For this review, take the finished solid that the model builds, in its own axes (mm). Face numbers are marked on the shaded views. A direction names the side the tool comes from. Round coordinates to 2 decimals unless told otherwise and drop trailing zeros. Order: outer loops, then holes, each group sorted by start corner. A loop starts at its lowest first (then second) coordinate and runs counter-clockwise, first axis right, second up. Notation, with made-up numbers: M 48.25,-11.5 L 104.25,-11.5 A25 cw 104.25,3.5 Z; hole C 18.25,24 d8. An arc over 180 degrees is marked long. Answer as a JSON object with one key per item and string values.
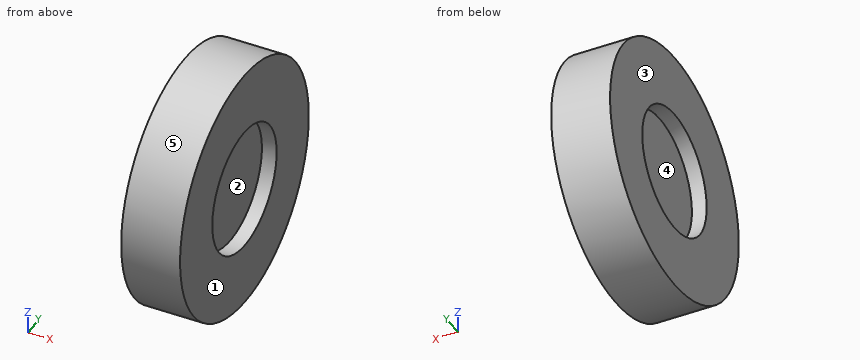
from build123d import *

# Parameters (mm, degrees)
SKETCH_1_W = 3
SKETCH_1_H = 6.35
SKETCH_4_W = 6
SKETCH_4_H = 6.35


with BuildPart() as part:
    # 草图1 → 旋转2 (revolve)
    with BuildSketch(Plane.XY, mode=Mode.PRIVATE) as revolve_2_sk:
        with Locations((0, 3.175)):
            Rectangle(SKETCH_1_W, SKETCH_1_H)
    revolve(revolve_2_sk.sketch.rotate(Axis((-1.5, 0, 0), (1, 0, 0)), 90), axis=Axis((-1.5, 0, 0), (1, 0, 0)))  # turned: the seam where the file's is

    # 草图4 → 旋转3 (revolve)
    with BuildSketch(Plane.XY, mode=Mode.PRIVATE) as revolve_3_sk:
        with Locations((0, 9.525)):
            Rectangle(SKETCH_4_W, SKETCH_4_H)
    revolve(revolve_3_sk.sketch.rotate(Axis((-1.614212419, 0, 0), (1, 0, 0)), 90), axis=Axis((-1.614212419, 0, 0), (1, 0, 0)))  # turned: the seam where the file's is


solid = part.part
1) Machinability: for the marked faces 1 and 2, which of the approach directions +Z, -Z, +X, -X, +Y, -Y give a long, thin tool a straight path to every point of the face, cutting with its end or side? Answer none if there is none.
Geometry check:
{"face 1": "+Z, -Z, +X, +Y, -Y", "face 2": "+X"}
2) Mouldability with a two-part tool opening along Y and no side actions: class the marked faces 3, 4 and 5 as +Y half, -Y half, draft (parallel to the pull), parting line (faces both ways), or undercut.
Geometry check:
{"face 3": "draft", "face 4": "undercut", "face 5": "parting line"}
3) Add section C-C on z = 8. State the section outline as (x, y) points.
Geometry check:
{"outline": "M -3,-9.86 L 3,-9.86 L 3,9.86 L -3,9.86 Z"}
4) Add section B-B on z = -1.5. State the section outline as (x, y) points.
Geometry check:
{"outline": "M -3,-12.61 L 3,-12.61 L 3,-6.17 L 1.5,-6.17 L 1.5,6.17 L 3,6.17 L 3,12.61 L -3,12.61 L -3,6.17 L -1.5,6.17 L -1.5,-6.17 L -3,-6.17 Z"}
5) For L1, parallel to Y at x = 2.55, z = 0; L2, parallel to X at y = 1.75, z = 5.5; L3, parallel to Z at x = 1.6, y = 11, list the stretches that pass through material, from the lowest coordinate up.
Geometry check:
{"L1": "y = -12.7 to -6.35, 6.35 to 12.7", "L2": "x = -1.5 to 1.5", "L3": "z = -6.35 to 6.35"}
6) Add section A-A on y = 0. State the section outline as (x, z) points, and give its area (3 significant figures).
Geometry check:
{"outline": "M -3,-12.7 L 3,-12.7 L 3,-6.35 L 1.5,-6.35 L 1.5,6.35 L 3,6.35 L 3,12.7 L -3,12.7 L -3,6.35 L -1.5,6.35 L -1.5,-6.35 L -3,-6.35 Z", "area": "114 mm²"}
7) Insertion check: P1, Ø10, axis at y = 0, z = 0, coming from the +X side; P2, Ø3, axis at x = 0, z = -2.5, coming from the -Y side; P3, Ø2, axis at x = -2, y = 7, coming from the -Z side. Each pin has a flat end and moves straight along its axis. Give the tip position at first contact, or say it passes through.
Geometry check:
{"P1": "stops at x = 1.5", "P2": "stops at y = -12.66", "P3": "stops at z = -11.19"}
